Model file for the job. Use its own axes, mm. Face numbers are marked on the shaded views. A direction names the side the tool comes from. Coordinates: 2 decimals unless noted, no trailing zeros. Order: outer loops, then holes, each group sorted by start corner. A loop starts at its lowest first (then second) coordinate and runs counter-clockwise, first axis right, second up. Notation, with made-up numbers: M 36,-11 L 58,-11 A30 ccw 58,19 Z; hole C 9,34 d9. An arc over 180 degrees is marked long. Return JSON: item names as keys, results as strings.
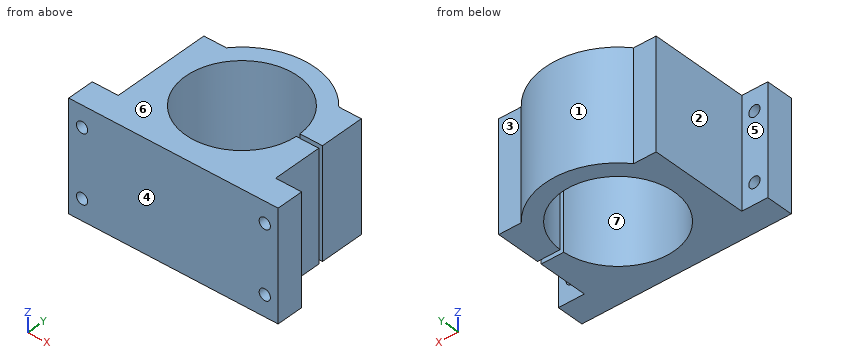
```python
from build123d import *

# Parameters (mm, degrees)
BOSS_EXTRUDE1_DEPTH = 78
SKETCH2_R           = 4
CUT_EXTRUDE1_DEPTH  = 200.872459333


with BuildPart() as part:
    # Sketch1 → Boss-Extrude1 (new body)
    with BuildSketch(Plane.XY):
        with BuildLine():
            Line((0, 19.226495452), (18.5, 19.226495452))
            Line((18.5, 19.226495452), (18.5, 89.226495452))
            Line((18.5, 89.226495452), (34.5, 89.226495452))
            ThreePointArc((34.5, 89.226495452), (74.5, 108), (114.5, 89.226495452))
            Line((114.5, 89.226495452), (130.5, 89.226495452))
            Line((130.5, 89.226495452), (130.5, 57.5))
            Line((130.5, 57.5), (114.471865105, 57.5))
            ThreePointArc((114.471865105, 57.5), (34.5, 56), (114.471865105, 54.5))
            Line((114.471865105, 54.5), (130.5, 54.5))
            Line((130.5, 54.5), (130.5, 19.226495452))
            Line((130.5, 19.226495452), (149, 19.226495452))
            Line((149, 19.226495452), (149, 0))
            Line((149, 0), (0, 0))
            Line((0, 0), (0, 19.226495452))
        make_face()
    extrude(amount=BOSS_EXTRUDE1_DEPTH)

    # Sketch2 → Cut-Extrude1 (cut, through all)
    with BuildSketch(Plane.XZ):
        with Locations((9.5, 63)):
            Circle(SKETCH2_R)
        with Locations((139.5, 63)):
            Circle(SKETCH2_R)
        with Locations((9.5, 15)):
            Circle(SKETCH2_R)
        with Locations((139.5, 15)):
            Circle(SKETCH2_R)
    extrude(amount=-CUT_EXTRUDE1_DEPTH, mode=Mode.SUBTRACT)


solid = part.part
```
Item 1: Saw through at A-A (z = 15). Write the cut outline in (x, y), and give its area (3 significant figures).
Check result:
{"outline": "M 0,0 L 5.5,0 L 5.5,19.23 L 0,19.23 Z; M 13.5,0 L 135.5,0 L 135.5,19.23 L 130.5,19.23 L 130.5,54.5 L 114.47,54.5 A40 cw long 114.47,57.5 L 130.5,57.5 L 130.5,89.23 L 114.5,89.23 A52 ccw 34.5,89.23 L 18.5,89.23 L 18.5,19.23 L 13.5,19.23 Z; M 143.5,0 L 149,0 L 149,19.23 L 143.5,19.23 Z", "area": "6,370 mm2"}
Item 2: Pull direction Y, two halves, no side cores. Call the marked faces 4, 5, 6 and 7: +Y half, -Y half, draft (parallel to the pull), parting line (faces both ways), or undercut.
Check result:
{"face 4": "-Y half", "face 5": "+Y half", "face 6": "draft", "face 7": "undercut"}
Item 3: Saw through at C-C (x = 9.5). Write the cut outline in (y, z), and give its area (3 significant figures).
Check result:
{"outline": "M 0,0 L 19.23,0 L 19.23,11 L 0,11 Z; M 0,19 L 19.23,19 L 19.23,59 L 0,59 Z; M 0,67 L 19.23,67 L 19.23,78 L 0,78 Z", "area": "1,190 mm2"}
Item 4: Wall check: line 1 (Z direction, x = 9.5, y = 14.75); line 2 (X direction, y = 8, z = 63.5); line 3 (Y direction, x = 127.5, z = 23). Give the ranges that are in metal, low to high.
Check result:
{"line 1": "z = 0 to 11, 19 to 59, 67 to 78", "line 2": "x = 0 to 5.53, 13.47 to 135.53, 143.47 to 149", "line 3": "y = 0 to 54.5, 57.5 to 89.23"}
Item 5: 3-axis set-ups, long thin cutter, end or side, ignore diameter. For the marked faces 1, 2 and 3: which of +Z, -Z, +X, -X, +Y, -Y reach the whole face in a straight line?
Check result:
{"face 1": "+Z, -Z, +Y", "face 2": "+Z, -Z, -X, +Y", "face 3": "+Z, -Z, +X, +Y"}
Item 6: Drop flat-ended pins along their axis: pin 1 Ø15 at (x, z) = (142.5, 38) entering from +Y; pin 2 Ø2 at (y, z) = (58, 50.5) entering from +X; pin 3 Ø7 at (x, z) = (139.5, 15) entering from -Y; pin 4 Ø2 at (y, z) = (76, 15) entering from -X. Give the stop position or say it passes through.
Check result:
{"pin 1": "stops at y = 19.23", "pin 2": "stops at x = 130.5", "pin 3": "passes through", "pin 4": "stops at x = 18.5"}
Item 7: Saw through at B-B (x = 74.5). Write the cut outline in (y, z), and give its area (3 significant figures).
Check result:
{"outline": "M 0,0 L 16,0 L 16,78 L 0,78 Z; M 96,0 L 108,0 L 108,78 L 96,78 Z", "area": "2,180 mm2"}
Item 8: Saw through at D-D (y = 79). Write the cut outline in (x, z).
Check result:
{"outline": "M 18.5,0 L 41.77,0 L 41.77,78 L 18.5,78 Z; M 107.23,0 L 130.5,0 L 130.5,78 L 107.23,78 Z"}
